The listing builds one solid part. Answer for the finished solid, in the listing's coordinates (mm). A direction names the side the tool comes from. Round coordinates to 2 decimals unless told otherwise and drop trailing zeros. Write each loop counter-clockwise with the first axis right and the second up, starting at its lowest first coordinate (ties: lowest second). Pieces come first, ordered by that corner, then holes. Notation, with made-up numbers: M 55.5,-32.75 L 103.5,-32.75 A26 ccw 103.5,-13.75 Z; hole C -32.75,-21.75 d2. An arc over 180 degrees is marked long. Put each result on its own line as item: value. Start each with the question number.
```python
from build123d import *

# Parameters (mm, degrees)
BOSS_EXTRUDE1_DEPTH = 3.8
SHELL1_START        = -21
SHELL1_OUTLINE_W    = 10.25
SHELL1_OUTLINE_H    = 3.5
SHELL1_DEPTH        = 20.7
SHELL1_START_2      = -19.893320937
SHELL1_2_OUTLINE_W  = 1.75
SHELL1_2_OUTLINE_H  = 3.5
SHELL1_2_DEPTH      = 3.893320937
BOSS_EXTRUDE2_DEPTH = 3.2
FILLET1_R           = 1.5
FILLET2_R           = 1.5
SKETCH4_W           = 5.1
SKETCH4_H           = 0.3
BOSS_EXTRUDE3_DEPTH = 4.8
FILLET3_R           = 0.2
SKETCH5_R           = 1.028757753
CUT_EXTRUDE1_DEPTH  = 4.8
FILLET4_R           = 0.2
FILLET5_R           = 0.2
FILLET6_START       = -5
FILLET6_DEPTH       = 10
FILLET6_START_2     = -19.893320937
FILLET6_2_DEPTH     = 13.893320937


with BuildPart() as part:
    # Sketch2 → Boss-Extrude1 (new body)
    with BuildSketch(Plane(origin=(0, 0, 0), x_dir=(1, 0, 0), z_dir=(0, 1, 0))):
        with BuildLine():
            Line((0, 0), (-3.75, 0))
            Line((-3.75, 0), (-10.55, 7))
            Line((-10.55, 7), (-10.55, 16))
            ThreePointArc((-10.55, 16), (-8.229026759, 19.561694912), (-4.03336762, 18.876835935))
            ThreePointArc((-4.03336762, 18.876835935), (-2.162785983, 17.71835226), (0, 17.313980062))
            Line((0, 17.313980062), (0, 0))
        make_face()
        with BuildLine():
            Line((-7.1, 13.769163671), (-7.1, 17.313980062))
            Line((-7.1, 17.313980062), (-3.9, 17.313980062))
            Line((-3.9, 17.313980062), (-3.9, 13.769163671))
            ThreePointArc((-3.9, 13.769163671), (-5.5, 8.013980062), (-7.1, 13.769163671))
        make_face(mode=Mode.SUBTRACT)
    extrude(amount=BOSS_EXTRUDE1_DEPTH)

    # Shell1: read off the stored shape, not the designer's step
    # Shell1 outline → Shell1 (cut)
    with BuildSketch(Plane.XY.offset(SHELL1_START)):
        with Locations((-5.125, 1.75)):
            Rectangle(SHELL1_OUTLINE_W, SHELL1_OUTLINE_H)
    extrude(amount=SHELL1_DEPTH, mode=Mode.SUBTRACT)

    # Shell1 2 outline → Shell1 2 (cut)
    with BuildSketch(Plane.XY.offset(SHELL1_START_2)):
        with Locations((-11.125, 1.75)):
            Rectangle(SHELL1_2_OUTLINE_W, SHELL1_2_OUTLINE_H)
    extrude(amount=SHELL1_2_DEPTH, mode=Mode.SUBTRACT)

    # Sketch3 → Boss-Extrude2 (add)
    with BuildSketch(Plane(origin=(-7.1, 0, 0), x_dir=(0, 0, -1), z_dir=(1, 0, 0))):
        Polygon((17.313980062, 3.5), (11.640356881, 1), (9.614191522, 1), (9.614191522, 1.3), (11.640356881, 1.3), (17.313980062, 3.8), align=None)
    extrude(amount=BOSS_EXTRUDE2_DEPTH)

    # Fillet1
    fillet1_edges = [part.edges().sort_by_distance(p)[0] for p in [
        (-3.9, 1.15, -9.614191522),
        (-7.1, 1.15, -9.614191522),
    ]]
    fillet(fillet1_edges, radius=FILLET1_R)

    # Fillet2
    fillet2_edges = [part.edges().sort_by_distance(p)[0] for p in [
        (-5.5, 3.8, -17.313980062),
        (-5.5, 3.5, -17.313980062),
    ]]
    fillet(fillet2_edges, radius=FILLET2_R)

    # Sketch4 → Boss-Extrude3 (add)
    with BuildSketch(Plane.ZY.offset(10.55)):
        with Locations((-11.05, 0.15)):
            Rectangle(SKETCH4_W, SKETCH4_H)
    extrude(amount=BOSS_EXTRUDE3_DEPTH)

    # Fillet3
    fillet3_edges = [part.edges().sort_by_distance(p)[0] for p in [
        (-10.55, 0.3, -11.05),
    ]]
    fillet(fillet3_edges, radius=FILLET3_R)

    # Sketch5 → Cut-Extrude1 (cut)
    with BuildSketch(Plane(origin=(0, 0.3, 0), x_dir=(1, 0, 0), z_dir=(0, 1, 0))):
        with Locations(Location((-12.85, 11, 0), (0, 0, 270))):
            Circle(SKETCH5_R)
    extrude(amount=-CUT_EXTRUDE1_DEPTH, mode=Mode.SUBTRACT)

    # Fillet4
    fillet4_edges = [part.edges().sort_by_distance(p)[0] for p in [
        (-10.25, 0, -11.345588235),
    ]]
    fillet(fillet4_edges, radius=FILLET4_R)

    # Mirror1: part across plane


with BuildPart() as part_1:
    add(part.part)
    add(part.part.mirror(Plane(origin=(0, 3.8, -17.313980062), x_dir=(0, 0, 1), z_dir=(-1, 0, 0))))

    # Fillet5
    fillet5_edges = [part_1.edges().sort_by_distance(p)[0] for p in [
        (10.25, 3.5, -11.345588235),
        (-10.25, 3.5, -11.345588235),
        (0, 3.5, -0.3),
    ]]
    fillet(fillet5_edges, radius=FILLET5_R)

    # Fillet6: read off the stored shape, not the designer's step
    # Fillet6 outline → Fillet6 (cut)
    with BuildSketch(Plane.YZ.offset(FILLET6_START)):
        with BuildLine():
            ThreePointArc((3.5, 0), (3.712132034, -0.087867966), (3.8, -0.3))
            Line((3.8, -0.3), (3.8, 0))
            Line((3.8, 0), (3.5, 0))
        make_face()
    extrude(amount=FILLET6_DEPTH, mode=Mode.SUBTRACT)

    # Fillet6 2 outline → Fillet6 2 (cut)
    with BuildSketch(Plane.XY.offset(FILLET6_START_2)):
        with BuildLine():
            Line((10.55, 3.8), (10.25, 3.8))
            ThreePointArc((10.25, 3.8), (10.462132034, 3.712132034), (10.55, 3.5))
            Line((10.55, 3.5), (10.55, 3.8))
        make_face()
        with BuildLine():
            ThreePointArc((-10.55, 3.5), (-10.462132034, 3.712132034), (-10.25, 3.8))
            Line((-10.25, 3.8), (-10.55, 3.8))
            Line((-10.55, 3.8), (-10.55, 3.5))
        make_face()
    extrude(amount=FILLET6_2_DEPTH, mode=Mode.SUBTRACT)


solid = part_1.part
```
Item 1: Section D-D (x = 5) is taken. Give the vertices of the cut face in (y, z).
Item 2: Section A-A (x = 12.85) is taken. Give the vertices of the cut face in (y, z), and give its area (3 significant figures).
Item 3: Determine the mould class of faces 4 (the flat face through (14.04, 0.3, -11.09)), 5 (the flat face through (0, 2, 0)), 6 (the cylindrical face through (-11.83, 0.15, -11.13)) for opening direction Z: released by +Z, released by -Z, zero draft, split by the parting line, or undercut.
Item 4: Section C-C (y = 1.65) is taken. Give the vertices of the cut face in (x, z), and give its area (3 significant figures).
Item 5: Section B-B (z = -15) is taken. Count the separate pieces of the cut face and the enclosed holes in it, and give its area (3 significant figures).
Item 6: Flat-ended cylindrical pins translate along their axes: pin 1 (1.6 mm diameter, centred on x = 5.5, z = -11, fed in from +Y); pin 2 (1.4 mm diameter, centred on x = 13.5, z = -11.5, fed in from +Y); pin 3 (0.6 mm diameter, centred on x = 6, z = -10.5, fed in from -Y). Find the tip coordinate at first contact, or state that the pin passes through.
Item 7: Which of the six approach directions +Z, -Z, +X, -X, +Y, -Y give full straight-line access (tool end or side, diameter ignored) to faces 1 (the flat face through (-14.04, 0.3, -11.09)), 2 (the flat face through (10.25, 2, -11)), 3 (the flat face through (0, 3.8, -10))?
Item 8: Consider line 1 along Z through (x, y) = (12.85, 0.1); line 2 along Z through (x, y) = (-1, 3.05); line 3 along X through (y, z) = (0.1, -11). Determine where each line is inside the solid, lowest interval first. Write a range as [from, to].
Output values:
1. outline: M 1,-11.64 L 3.37,-17.02 A1.5 cw 3.5,-17.63 L 3.5,-19.52 L 3.8,-19.52 L 3.8,-17.63 A1.5 ccw 3.67,-17.02 L 1.3,-11.64 L 1.3,-9.67 L 1,-9.67 Z; M 3.5,-8.05 L 3.8,-8.05 L 3.8,-1.29 L 3.5,-1.29 Z
2. outline: M 0,-13.6 L 0.3,-13.6 L 0.3,-12.03 L 0,-12.03 Z; M 0,-9.97 L 0.3,-9.97 L 0.3,-8.5 L 0,-8.5 Z
2. area: 0.913 mm^2
3. face 4: zero draft
3. face 5: released by +Z
3. face 6: undercut
4. outline: M -10.55,-16 L -10.25,-16 L -10.25,-6.69 L -10.55,-7 Z; M -7.1,-13.12 L -3.9,-13.12 L -3.9,-12.43 L -7.1,-12.43 Z; M -4.04,-0.3 L 4.04,-0.3 L 3.75,0 L -3.75,0 Z; M 3.9,-13.12 L 7.1,-13.12 L 7.1,-12.43 L 3.9,-12.43 Z; M 10.25,-16 L 10.55,-16 L 10.55,-7 L 10.25,-6.69 Z
4. area: 12.2 mm^2
5. separate pieces: 5
5. enclosed holes: 0
5. area: 8.39 mm^2
6. pin 1: stops at y = 1.37
6. pin 2: stops at y = 0.3
6. pin 3: stops at y = 1
7. face 1: +Z, -Z, -X, +Y
7. face 2: +Z, -Z, -Y
7. face 3: +Z, -Z, +X, -X, +Y
8. line 1: z = [-13.6, -12.03], [-9.97, -8.5]
8. line 2: z = [-0.3, 0]
8. line 3: x = [-15.35, -13.88], [-11.82, -10.28], [10.28, 11.82], [13.88, 15.35]
